For this review, take the finished solid that the model builds, in its own axes (mm). Face numbers are marked on the shaded views. Round coordinates to 2 decimals unless told otherwise and drop trailing zeros. Write each loop counter-clockwise with the first axis right and the second up, starting at its lowest first coordinate (ties: lowest second). Pieces come first, ordered by that corner, then holes. Notation, with made-up numbers: M 32.25,16.5 L 40.25,16.5 A21 cw 40.25,42.5 Z; hole C 82.25,-5.5 d2. An arc over 180 degrees is marked long. Write each question's results on one line, items separated by ' | '. Start each with the question number.
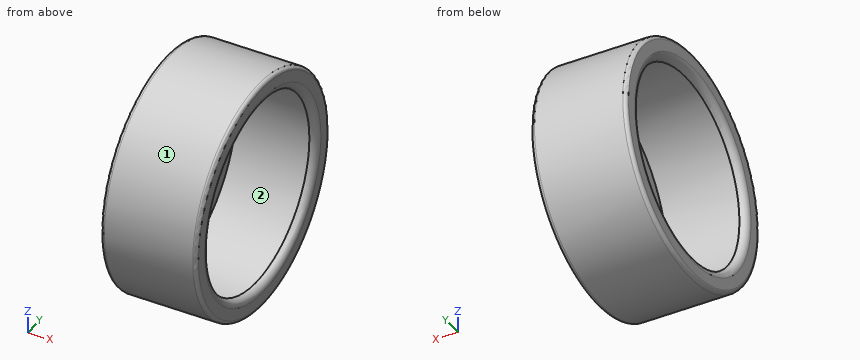
```python
from build123d import *

# Parameters (mm, degrees)
SKETCH1_R           = 32
SKETCH1_R_2         = 26
BOSS_EXTRUDE1_DEPTH = 26
FILLET1_R           = 1
FILLET2_R           = 2
SHELL1_START        = 2
SHELL1_OUTLINE_R    = 30
SHELL1_OUTLINE_R_2  = 26
SHELL1_DEPTH        = 22


# Read off the part's stored shape, not the designer's step: Shell1
with BuildPart() as part:
    # Sketch1 → Boss-Extrude1 (new body)
    with BuildSketch(Plane(origin=(0, 0, 0), x_dir=(0, 0, -1), z_dir=(1, 0, 0))):
        with Locations(Location((0, 0, 0), (0, 0, 180))):
            Circle(SKETCH1_R)
        with Locations(Location((0, 0, 0), (0, 0, 180))):
            Circle(SKETCH1_R_2, mode=Mode.SUBTRACT)
    extrude(amount=BOSS_EXTRUDE1_DEPTH)

    # Fillet1
    fillet1_edges = [part.edges().sort_by_distance(p)[0] for p in [
        (0, 0, -32),
        (26, 0, -32),
    ]]
    fillet(fillet1_edges, radius=FILLET1_R)

    # Fillet2
    fillet2_edges = [part.edges().sort_by_distance(p)[0] for p in [
        (0, 0, -26),
        (26, 0, -26),
    ]]
    fillet(fillet2_edges, radius=FILLET2_R)

    # Shell1 outline → Shell1 (cut)
    with BuildSketch(Plane.YZ.offset(SHELL1_START)):
        Circle(SHELL1_OUTLINE_R)
        Circle(SHELL1_OUTLINE_R_2, mode=Mode.SUBTRACT)
    extrude(amount=SHELL1_DEPTH, mode=Mode.SUBTRACT)


solid = part.part
```
Item 1: For probe 1 along Z at (x, y) = (15.25, 0.5); probe 2 along X at (y, z) = (21, -21), list the stretches that pass through material, from the lowest coordinate up.
Item 2: We need section C-C on x = 21. State the section outline as (y, z) points, then the cut area to 3 significant figures.
Item 3: We need section A-A on z = 0. State the section outline as (x, y) points, then the cut area to 3 significant figures.
Item 4: Insertion check: P1, Ø6, axis at x = 21, z = -12.5, coming from the -Y side; P2, Ø8, axis at y = -1.5, z = 24.5, coming from the -X side; P3, Ø2, axis at x = 19, z = 21, coming from the +Y side; P4, Ø1.5, axis at x = 6, y = 7, coming from the +Z side. Each pin has a flat end and moves straight along its axis. Give the tip position at first contact, or say it passes through.
Item 5: Mouldability with a two-part tool opening along Y and no side actions: class the marked faces 1 and 2 as pulls with the +Y half, pulls with the -Y half, needs draft (parallel to the pull), parting line crosses it, or undercut.
Numbers:
1) probe 1: z = -32 to -30, 30 to 32 | probe 2: x = 0 to 2, 24 to 26
2) outline: C 0,0 d64; hole C 0,0 d60 | area: 390 mm^2
3) outline: M 0,-31 A1 ccw 1,-32 L 25,-32 A1 ccw 26,-31 L 26,-28 A2 ccw 24,-26 L 24,-30 L 2,-30 L 2,-26 A2 ccw 0,-28 Z; M 0,28 A2 ccw 2,26 L 2,30 L 24,30 L 24,26 A2 ccw 26,28 L 26,31 A1 ccw 25,32 L 1,32 A1 ccw 0,31 Z | area: 132 mm^2
4) P1: stops at y = -30.56 | P2: stops at x = 0 | P3: stops at y = 24.98 | P4: stops at z = 31.38
5) face 1: parting line crosses it | face 2: undercut
